Build history of the part. All positions in model axes, mm. Face numbers are marked on the shaded views. A direction names the side the tool comes from. Coordinates: 2 decimals unless noted, no trailing zeros. Order: outer loops, then holes, each group sorted by start corner. A loop starts at its lowest first (then second) coordinate and runs counter-clockwise, first axis right, second up. Notation, with made-up numbers: M 14,0 L 64,0 A26 ccw 64,34 Z; hole C -10,70 d4. An arc over 180 degrees is marked long. Write item = value, one per line. Start each with the question number.
Q1. 3-axis set-ups, long thin cutter, end or side, ignore diameter. For the marked faces 5, 6 and 7: which of +Z, -Z, +X, -X, +Y, -Y reach the whole face in a straight line?
Q2. Band-saw the part on B-B on y = -14. State how many separate pieces and enclosed holes the cut face has, plus the area to 3 significant figures.
Q3. Pull direction X, two halves, no side cores. Call the marked faces 1, 2, 3 and 4: released by +X, released by -X, zero draft, split by the parting line, or undercut.
Q4. Band-saw the part on A-A on x = -30. Write the cut outline in (y, z), plus the area to 3 significant figures.
Q5. Drill centre lines: probe 1 along Z at (x, y) = (86, -3); probe 2 along X at (y, z) = (-2.5, -2); probe 3 along Y at (x, z) = (12, -3.75). Where is each one in solid material? Low to high.
Q6. Pin check, flat tips, straight feed: P1, Ø2.5, axis at y = -6.5, z = -1, coming from the -X side; P2, Ø3, axis at x = -28.5, z = -5.5, coming from the +Y side; P3, Ø10, axis at y = -6, z = 7.5, coming from the -X side; P4, Ø3, axis at x = -86, z = 0, coming from the +Y side. Stop position of each tip, or through.
```python
from build123d import *

# Parameters (mm, degrees)
PAD_DEPTH       = 10
SKETCH001_R     = 2.7
POCKET_DEPTH    = 40
SKETCH002_R     = 5
POCKET001_DEPTH = 24
POCKET001_TAPER = -5
FILLET_R        = 9
FILLET001_R     = 15
CHAMFER_SIZE    = 0.6
FILLET002_R     = 3
FILLET003_R     = 5


with BuildPart() as part:
    # Sketch (on XY_Plane of Origin) → Pad (new body, symmetric)
    with BuildSketch(Plane.XY):
        Polygon((71, 0), (71, -15), (56, -30), (0, -30), (0, -50), (56, -50), (91, -23.284271), (101, 0), align=None)
    extrude(amount=PAD_DEPTH, both=True)

    # Sketch001 (on Face8 of Pad) → Pocket (cut)
    with BuildSketch(Plane(origin=(0, 0, 0), x_dir=(-1, 0, 0), z_dir=(0, 1, 0))):
        with Locations((-86, 0)):
            Circle(SKETCH001_R)
    extrude(amount=-POCKET_DEPTH, mode=Mode.SUBTRACT)

    # Sketch002 (on Face2 of Pocket) → Pocket001 (cut)
    with BuildSketch(Plane(origin=(0, -10, 0), x_dir=(-1, 0, 0), z_dir=(0, 1, 0))):
        with Locations((-86, 0)):
            Circle(SKETCH002_R)
    extrude(amount=-POCKET001_DEPTH, taper=POCKET001_TAPER, mode=Mode.SUBTRACT)

    # Fillet
    fillet_edges = [part.edges().sort_by_distance(p)[0] for p in [
        (91, -23.284271, 6.800902),
        (91, -23.284271, -6.800902),
    ]]
    fillet(fillet_edges, radius=FILLET_R)

    # Fillet001
    fillet001_edges = [part.edges().sort_by_distance(p)[0] for p in [
        (56, -50, 0),
        (56, -30, 0),
        (71, -15, 0),
    ]]
    fillet(fillet001_edges, radius=FILLET001_R)

    # Chamfer
    chamfer_edges = [part.edges().sort_by_distance(p)[0] for p in [
        (88.7, 0, 0),
    ]]
    chamfer(chamfer_edges, length=CHAMFER_SIZE)

    # Mirrored: part across YZ


with BuildPart() as part_1:
    add(part.part)
    add(part.part.mirror(Plane.YZ))

    # Fillet002
    fillet002_edges = [part_1.edges().sort_by_distance(p)[0] for p in [
        (0, -50, 10),
        (0, -50, -10),
    ]]
    fillet(fillet002_edges, radius=FILLET002_R)

    # Fillet003
    fillet003_edges = [part_1.edges().sort_by_distance(p)[0] for p in [
        (0, -30, 10),
        (0, -30, -10),
    ]]
    fillet(fillet003_edges, radius=FILLET003_R)


solid = part_1.part
```
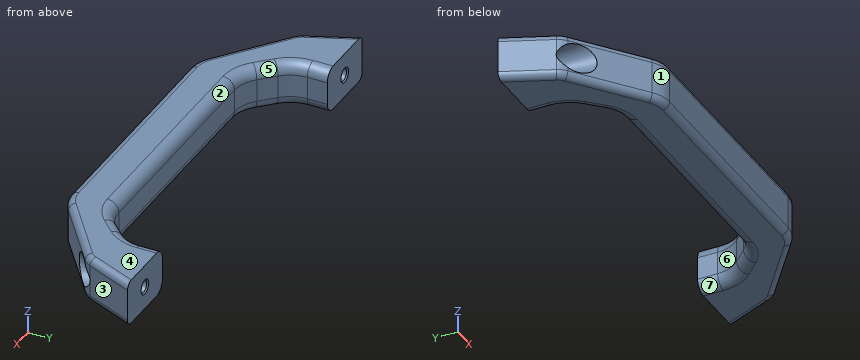
Recorded:
q1.face_5 = +Z, +Y
q1.face_6 = +Z, -Z, +Y
q1.face_7 = -Z, +Y
q2.separate_pieces = 2
q2.enclosed_holes = 2
q2.area = 786 mm2
q3.face_1 = released by -X
q3.face_2 = undercut
q3.face_3 = released by +X
q3.face_4 = zero draft
q4.outline = M -50,-7 A3 ccw -47,-10 L -35,-10 A5 ccw -30,-5 L -30,5 A5 ccw -35,10 L -47,10 A3 ccw -50,7 Z
q4.area = 385 mm2
q5.probe_1 = -10 to -2.7, 2.7 to 10
q5.probe_2 = -99.93 to -87.81, -84.19 to -71, 71 to 84.19, 87.81 to 99.93
q5.probe_3 = -50 to -30
q6.P1 = -98.75
q6.P2 = -30
q6.P3 = -100.56
q6.P4 = through
